from build123d import *

# Parameters (mm, degrees)
SKETCH1_R             = 1.5
BOSS_EXTRUDE1_DEPTH   = 3
SKETCH1_R_2           = 3
BOSS_EXTRUDE1_2_DEPTH = 3
EXTRUDE_THIN1_DEPTH   = 3
BOSS_EXTRUDE2_DEPTH   = 3
FILLET1_R             = 10
FILLET2_R             = 10
FILLET3_R             = 5
CUT_EXTRUDE2_DEPTH    = 3
CHAMFER1_SIZE         = 0.25
FILLET4_SIZE          = 0.5


with BuildPart() as part:
    # Sketch1 → Boss-Extrude1 (new body)
    with BuildSketch(Plane.XY.offset(5)):
        with BuildLine():
            ThreePointArc((109.185458354, -4.000646729), (108.5228767, -5.038603319), (108.360025672, -6.259196566))
            ThreePointArc((108.360025672, -6.259196566), (108.310958913, -9.715379327), (107.5808738, -13.093926729))
            ThreePointArc((107.5808738, -13.093926729), (110.294106049, -17.011846795), (113.365194477, -13.367653777))
            ThreePointArc((113.365194477, -13.367653777), (113.140936636, -10.174222756), (113.854520762, -7.053471091))
            ThreePointArc((113.854520762, -7.053471091), (112.759359915, -3.631536319), (109.185458354, -4.000646729))
        make_face()
        with Locations((111.199707869, -6.016905367)):
            Circle(SKETCH1_R, mode=Mode.SUBTRACT)
        with Locations((110.435914095, -14.015200256)):
            Circle(SKETCH1_R, mode=Mode.SUBTRACT)
    extrude(amount=BOSS_EXTRUDE1_DEPTH)



with BuildPart() as body_2:
    # Sketch1 → Boss-Extrude1 2 (new body)
    with BuildSketch(Plane.XY.offset(5)):
        with Locations((39, 9.5)):
            Circle(SKETCH1_R_2)
        with Locations((39, 9.5)):
            Circle(SKETCH1_R, mode=Mode.SUBTRACT)
    extrude(amount=BOSS_EXTRUDE1_2_DEPTH)


with BuildPart() as part_1:
    add(part.part)

    add(body_2.part)  # Extrude-Thin1 merges body 2
    # Sketch3 → Extrude-Thin1 (add)
    with BuildSketch(Plane.XY.offset(5)):
        with BuildLine():
            ThreePointArc((41.593001143, 9.173549984), (52.518716901, 11.608273697), (63.103455441, 7.966508408))
            ThreePointArc((63.103455441, 7.966508408), (67.496674945, 5.672669193), (72.321939964, 4.541787477))
            Line((72.321939964, 4.541787477), (94.785034536, 2.180821101))
            ThreePointArc((94.785034536, 2.180821101), (102.503244611, -0.298409767), (108.581874595, -5.661954302))
            Line((108.581874595, -5.661954302), (110.985068552, -3.8662208))
            ThreePointArc((110.985068552, -3.8662208), (103.98579607, 2.309662542), (95.098619926, 5.164386787))
            Line((95.098619926, 5.164386787), (72.635525354, 7.525353163))
            ThreePointArc((72.635525354, 7.525353163), (68.541425508, 8.484874068), (64.813903968, 10.431131266))
            ThreePointArc((64.813903968, 10.431131266), (52.686795037, 14.60356162), (40.169022902, 11.814058641))
            Line((40.169022902, 11.814058641), (41.593001143, 9.173549984))
        make_face()
    extrude(amount=EXTRUDE_THIN1_DEPTH)

    # Sketch4 → Boss-Extrude2 (add)
    with BuildSketch(Plane.XY.offset(8)):
        Polygon((71.8385125, 9.620139149), (90.734428512, 7.634098347), (90.002729269, 0.672445079), (71.106813257, 2.658485881), align=None)
        with BuildLine():
            Line((77.099325998, 7.05618881), (85.055501161, 6.219961104))
            ThreePointArc((85.055501161, 6.219961104), (86.390491309, 4.571385566), (84.741915771, 3.236395418))
            Line((84.741915771, 3.236395418), (76.785740608, 4.072623124))
            ThreePointArc((76.785740608, 4.072623124), (75.45075046, 5.721198662), (77.099325998, 7.05618881))
        make_face(mode=Mode.SUBTRACT)
    extrude(amount=-BOSS_EXTRUDE2_DEPTH)

    # Fillet1
    # the kernel refuses this fillet: 10 mm, written as the material it takes off along each edge
    with BuildSketch(Plane(origin=(90.002729269, 0.672445079, 23), x_dir=(0.10452846326752661, 0.9945218953682867, 0), z_dir=(0, 0, -1))) as fillet1_piece_1:
        with BuildLine():
            CenterArc((10, -6), FILLET1_R, 143.130102354, 36.869897646)
            Line((0, -6), (-0.2, -6))
            Line((-0.2, -6), (-0.2, 0))
            Line((-0.2, 0), (0, 0.2))
            ThreePointArc((0, 0.2), (1, 0.2), (1.84, 0.12))
            Line((1.84, 0.12), (2, 0))
        make_face()
    extrude(amount=33, mode=Mode.SUBTRACT)
    with BuildSketch(Plane(origin=(90.734428512, 7.634098347, 23), x_dir=(-0.10452846326775972, -0.9945218953682622, 0), z_dir=(0, 0, -1))) as fillet1_piece_2:
        with BuildLine():
            CenterArc((10, 6), FILLET1_R, 180, 36.869897646)
            Line((0, 6), (-0.2, 6))
            Line((-0.2, 6), (-0.2, 0))
            Line((-0.2, 0), (0, -0.2))
            ThreePointArc((0, -0.2), (1, -0.2), (1.84, -0.12))
            Line((1.84, -0.12), (2, 0))
        make_face()
    extrude(amount=33, mode=Mode.SUBTRACT)
    with BuildSketch(Plane(origin=(71.106813257, 2.658485881, 23.085820281), x_dir=(0.9945218953682746, -0.10452846326764255, 0), z_dir=(0, 0, -1))) as fillet1_piece_3:
        with BuildLine():
            CenterArc((6.034328112, -10), FILLET1_R, 90, 37.116152296)
            Line((0, -2.025861537), (-0.120686562, -1.866378767))
            ThreePointArc((-0.120686562, -1.866378767), (-0.2, -1.012930768), (-0.2, 0))
            Line((-0.2, 0), (0, 0.2))
            Line((0, 0.2), (6.034328112, 0.2))
            Line((6.034328112, 0.2), (6.034328112, 0))
        make_face()
    extrude(amount=33.171640562, mode=Mode.SUBTRACT)
    with BuildSketch(Plane(origin=(71.8385125, 9.620139149, 22.897832051), x_dir=(-0.10452846326748966, -0.9945218953682906, 0), z_dir=(0, 0, -1))) as fillet1_piece_4:
        with BuildLine():
            CenterArc((10, -5.95913282), FILLET1_R, 143.422234679, 36.577765321)
            Line((0, -5.95913282), (-0.2, -5.95913282))
            Line((-0.2, -5.95913282), (-0.2, 0))
            Line((-0.2, 0), (0, 0.2))
            ThreePointArc((0, 0.2), (0.984756046, 0.2), (1.808902334, 0.119182656))
            Line((1.808902334, 0.119182656), (1.969512093, 0))
        make_face()
    extrude(amount=32.795664101, mode=Mode.SUBTRACT)

    # Fillet2
    fillet2_edges = [part_1.edges().sort_by_distance(p)[0] for p in [
        (71.632642427, 7.66141625, 6.5),
        (90.525371585, 5.645054556, 6.5),
        (90.211786196, 2.66148887, 6.5),
        (71.31857345, 4.673249537, 6.5),
    ]]
    fillet(fillet2_edges, radius=FILLET2_R)

    # Fillet3
    fillet3_edges = [part_1.edges().sort_by_distance(p)[0] for p in [
        (108.409742984, -5.435015389, 6.5),
        (110.509408047, -3.251767729, 6.5),
        (41.997837089, 9.386101864, 6.5),
        (40.597330828, 12.039396429, 6.5),
    ]]
    fillet(fillet3_edges, radius=FILLET3_R)

    # Sketch4<2> → Cut-Extrude2 (cut)
    with BuildSketch(Plane.XY.offset(8)):
        with BuildLine():
            Line((77.099325998, 7.05618881), (85.055501161, 6.219961104))
            ThreePointArc((85.055501161, 6.219961104), (86.390491309, 4.571385566), (84.741915771, 3.236395418))
            Line((84.741915771, 3.236395418), (76.785740608, 4.072623124))
            ThreePointArc((76.785740608, 4.072623124), (75.45075046, 5.721198662), (77.099325998, 7.05618881))
        make_face()
    extrude(amount=-CUT_EXTRUDE2_DEPTH, mode=Mode.SUBTRACT)

    # Chamfer1
    chamfer1_edges = [part_1.edges().sort_by_distance(p)[0] for p in [
        (81.077413579, 6.638074957, 8),
        (86.390491309, 4.571385566, 5),
        (80.76382819, 3.654509271, 5),
        (75.45075046, 5.721198662, 5),
        (81.077413579, 6.638074957, 5),
        (75.45075046, 5.721198662, 8),
        (80.76382819, 3.654509271, 8),
        (86.390491309, 4.571385566, 8),
    ]]
    chamfer(chamfer1_edges, length=CHAMFER1_SIZE)

    # Fillet4
    fillet4_edges = [part_1.edges().sort_by_distance(p)[0] for p in [
        (80.571841293, 1.663671348, 5),
        (80.571841293, 1.663671348, 8),
        (81.266148853, 8.62925464, 8),
        (75.831843077, 9.0125273, 8),
        (86.285883658, 1.317701678, 8),
        (81.266148853, 8.62925464, 5),
        (74.746621894, 2.571133627, 5),
        (86.964648505, 7.775717809, 5),
        (74.746621894, 2.571133627, 8),
        (66.167237141, 6.222318503, 8),
        (66.167237141, 6.222318503, 5),
        (65.577546873, 9.931341027, 8),
        (65.577546873, 9.931341027, 5),
        (75.831843077, 9.0125273, 5),
        (86.285883658, 1.317701678, 5),
        (53.814375327, 14.513121306, 5),
        (86.964648505, 7.775717809, 8),
        (71.097481671, 4.489860289, 5),
        (54.015350868, 11.469337492, 8),
        (71.097481671, 4.489860289, 8),
        (70.068678069, 8.317079629, 5),
        (70.068678069, 8.317079629, 8),
        (90.66440994, 2.359315815, 8),
        (90.66440994, 2.359315815, 5),
        (91.030929726, 5.846518637, 8),
        (91.030929726, 5.846518637, 5),
        (93.849865119, 2.279111367, 8),
        (101.439573781, 0.26418945, 5),
        (101.439573781, 0.26418945, 8),
        (108.258346947, -10.132192641, 5),
        (108.258346947, -10.132192641, 8),
        (102.785056404, 2.945662756, 5),
        (102.785056404, 2.945662756, 8),
        (36.30994009, 8.172002379, 5),
        (36.30994009, 8.172002379, 8),
        (94.163450509, 5.262677053, 5),
        (108.019819848, -5.334888598, 8),
        (108.019819848, -5.334888598, 5),
        (110.407911183, -2.704163701, 8),
        (110.407911183, -2.704163701, 5),
        (42.773374787, 9.487301339, 8),
        (42.773374787, 9.487301339, 5),
        (40.865302991, 12.434666794, 8),
        (94.163450509, 5.262677053, 8),
        (40.865302991, 12.434666794, 5),
        (53.814375327, 14.513121306, 8),
        (54.015350868, 11.469337492, 5),
        (93.849865119, 2.279111367, 5),
        (113.710131038, -4.667729504, 5),
        (110.294106049, -17.011846795, 8),
        (113.710131038, -4.667729504, 8),
        (113.140936636, -10.174222756, 5),
        (110.294106049, -17.011846795, 5),
        (113.140936636, -10.174222756, 8),
    ]]
    chamfer(fillet4_edges, length=FILLET4_SIZE)


solid = part_1.part
Model file for the job. Use its own axes, mm. A direction names the side the tool comes from. Give positions to 0.01 mm unless a question says otherwise; leave off trailing zeros. Answer as CSV lines item,"result".
1. 3-axis set-ups, long thin cutter, end or side, ignore diameter. For faces 1 (the face through (66.122, 6.243, 6.486)), 2 (the face through (75.32, 5.7, 5.12)), 3 (the face through (108.264, -10.09, 6.486)): which of +Z, -Z, +X, -X, +Y, -Y reach the whole face in a straight line?
Responses:
face 1,"+Z, -Z, -Y"
face 2,"-Z"
face 3,"+Z, -Z, -X"
2. Two-plate mould, pull along Y, no slides. Class faces 4 (the face through (74.88, 2.84, 7.8)), 5 (the face through (80.9, 2.3, 8)), 6 (the face through (81.022, 6.644, 6.518)): +Y half, -Y half, draft (parallel to the pull), parting line (faces both ways), or undercut.
Responses:
face 4,"-Y half"
face 5,"draft"
face 6,"undercut"
3. Band-saw the part on A-A (z = 6.3). Count the separate pieces of the cut face and the enclosed holes in it, and give its area (3 significant figures).
Responses:
separate pieces,"1"
enclosed holes,"4"
area,"327 mm2"
4. Pin check, flat tips, straight feed: pin 1 (1.5 mm diameter, centred on x = 88, z = 6, fed in from -Y); pin 2 (3 mm diameter, centred on x = 70, y = 3, fed in from +Z); pin 3 (1.5 mm diameter, centred on y = -1, z = 6.5, fed in from +X); pin 4 (1 mm diameter, centred on x = 65.5, z = 7, fed in from +Y). Stop position of each tip, or through.
Responses:
pin 1,"stops at y = 1.48"
pin 2,"passes through"
pin 3,"stops at x = 109.19"
pin 4,"stops at y = 10.3"
5. Drill centre lines: L1, parallel to Y at x = 81.5, z = 7.15; L2, parallel to Y at x = 56.5, z = 7.4; L3, parallel to Y at x = 66, z = 6.45. Where is each one in solid material? Low to high. Write a range as [from, to].
Responses:
L1,"y = [1.57, 3.58], [6.59, 8.6]"
L2,"y = [10.99, 14.07]"
L3,"y = [6.3, 9.68]"
